Read the model definition and answer for the solid it produces. Units are mm, in the model's axes. A direction names the side the tool comes from. Coordinates: 2 decimals unless noted, no trailing zeros. Loops run counter-clockwise (first coordinate to the right, second up) from the corner with the lowest first, then second, coordinate; pieces in that order, holes last. Notation, with made-up numbers: (20.5, 86) -> (71.5, 86) arc R17 ccw to (71.5, 107) -> close; hole circle Ø9 at (-23, 43.5). An arc over 180 degrees is marked (long way). Answer as CSV lines item,"result".
```python
from build123d import *

# Parameters (mm, degrees)
SKETCH1_R           = 25.65
SKETCH1_R_2         = 16.9
SKETCH1_R_3         = 2.2
BOSS_EXTRUDE1_DEPTH = 3.1
SKETCH1_3_R         = 28.75
SKETCH1_3_R_2       = 25.65
BOSS_EXTRUDE2_DEPTH = 15
SKETCH2_R           = 2.2
BOSS_EXTRUDE4_DEPTH = 3.1


with BuildPart() as part:
    # Sketch1 → Boss-Extrude1 (new body)
    with BuildSketch(Plane(origin=(0, 0, 0), x_dir=(1, 0, 0), z_dir=(0, 1, 0))):
        Circle(SKETCH1_R)
        Circle(SKETCH1_R_2, mode=Mode.SUBTRACT)
        with Locations((0, 21.3)):
            Circle(SKETCH1_R_3, mode=Mode.SUBTRACT)
        with Locations((15.061374439, 15.061374439)):
            Circle(SKETCH1_R_3, mode=Mode.SUBTRACT)
        with Locations((21.3, 0)):
            Circle(SKETCH1_R_3, mode=Mode.SUBTRACT)
        with Locations((15.061374439, -15.061374439)):
            Circle(SKETCH1_R_3, mode=Mode.SUBTRACT)
        with Locations((0, -21.3)):
            Circle(SKETCH1_R_3, mode=Mode.SUBTRACT)
        with Locations((-15.061374439, -15.061374439)):
            Circle(SKETCH1_R_3, mode=Mode.SUBTRACT)
        with Locations((-21.3, 0)):
            Circle(SKETCH1_R_3, mode=Mode.SUBTRACT)
        with Locations((-15.061374439, 15.061374439)):
            Circle(SKETCH1_R_3, mode=Mode.SUBTRACT)
    extrude(amount=BOSS_EXTRUDE1_DEPTH)

    # Sketch1_3 → Boss-Extrude2 (add)
    with BuildSketch(Plane(origin=(0, 0, 0), x_dir=(1, 0, 0), z_dir=(0, 1, 0))):
        Circle(SKETCH1_3_R)
        Circle(SKETCH1_3_R_2, mode=Mode.SUBTRACT)
    extrude(amount=BOSS_EXTRUDE2_DEPTH)

    # Sketch2 → Boss-Extrude4 (add)
    with BuildSketch(Plane(origin=(0, 11.9, 0), x_dir=(1, 0, 0), z_dir=(0, 1, 0))):
        with BuildLine():
            ThreePointArc((25.65, 0), (25.555797131, 2.196299839), (25.273880469, 4.376467299))
            Line((25.273880469, 4.376467299), (20.845539906, 4.376467299))
            ThreePointArc((20.845539906, 4.376467299), (16.9, 0), (20.845539906, -4.376467299))
            Line((20.845539906, -4.376467299), (25.273880469, -4.376467299))
            ThreePointArc((25.273880469, -4.376467299), (25.555797131, -2.196299839), (25.65, 0))
        make_face()
        with Locations((21.3, 0)):
            Circle(SKETCH2_R, mode=Mode.SUBTRACT)
        with BuildLine():
            ThreePointArc((4.376467299, 25.273880469), (0, 25.65), (-4.376467299, 25.273880469))
            Line((-4.376467299, 25.273880469), (-4.376467299, 20.845539906))
            ThreePointArc((-4.376467299, 20.845539906), (0, 16.9), (4.376467299, 20.845539906))
            Line((4.376467299, 20.845539906), (4.376467299, 25.273880469))
        make_face()
        with Locations((0, 21.3)):
            Circle(SKETCH2_R, mode=Mode.SUBTRACT)
        with BuildLine():
            Line((-4.376467299, -20.845539906), (-4.376467299, -25.273880469))
            ThreePointArc((-4.376467299, -25.273880469), (0, -25.65), (4.376467299, -25.273880469))
            Line((4.376467299, -25.273880469), (4.376467299, -20.845539906))
            ThreePointArc((4.376467299, -20.845539906), (0, -16.9), (-4.376467299, -20.845539906))
        make_face()
        with Locations((0, -21.3)):
            Circle(SKETCH2_R, mode=Mode.SUBTRACT)
        with BuildLine():
            ThreePointArc((-20.845539906, -4.376467299), (-16.9, 0), (-20.845539906, 4.376467299))
            Line((-20.845539906, 4.376467299), (-25.273880469, 4.376467299))
            ThreePointArc((-25.273880469, 4.376467299), (-25.65, 0), (-25.273880469, -4.376467299))
            Line((-25.273880469, -4.376467299), (-20.845539906, -4.376467299))
        make_face()
        with Locations((-21.3, 0)):
            Circle(SKETCH2_R, mode=Mode.SUBTRACT)
    extrude(amount=BOSS_EXTRUDE4_DEPTH)


solid = part.part
```
Q1. Given pin 1 Ø5 at (x, y) = (6, 1.5) entering from +Z; pin 2 Ø1.5 at (x, y) = (-21, 10.5) entering from -Z; pin 3 Ø8 at (x, z) = (-3, -18) entering from +Y; pin 4 Ø2.5 at (y, z) = (14, 22.5) entering from +X, each flat-ended and moving along its own axis, determine where each tip first touches the part or whether it passes through.
Results:
pin 1,"stops at z = 28.54"
pin 2,"stops at z = -20.41"
pin 3,"stops at y = 15"
pin 4,"stops at x = 19.36"
Q2. For faces 1 (the face through (23, 13, -4.376)), 2 (the face through (17.16, 1.53, 14.4)), 3 (the face through (23, 11.9, 2)), determine the directions among +Z, -Z, +X, -X, +Y, -Y from which every point of the face is accessible in a straight line to the end or side of a thin tool.
Results:
face 1,"+Y"
face 2,"+Y, -Y"
face 3,"none"
Q3. A cutting plane is placed at D-D, the plane y = 5.75. Write down the section's boundary in (x, z).
Results:
outline,"circle Ø57.5 at (0, 0); hole circle Ø51.3 at (0, 0)"
Q4. For a pull along Y with two mould halves and no side action, classify faces 4 (the face through (-2.198, 1.528, -21.397)), 5 (the face through (23.694, 8.967, 9.824)), 6 (the face through (-17.2, 15, -0.1)) as pulls with the +Y half, pulls with the -Y half, needs draft (parallel to the pull), parting line crosses it, or undercut.
Results:
face 4,"needs draft"
face 5,"undercut"
face 6,"pulls with the +Y half"
Q5. Find the intervals of material crossed by probe 1 along Z at (x, y) = (0, 1.3); probe 2 along X at (y, z) = (13.05, 21.3), in increasing order. Write a range as [from, to].
Results:
probe 1,"z = [-28.75, -23.5], [-19.1, -16.9], [16.9, 19.1], [23.5, 28.75]"
probe 2,"x = [-19.31, -14.29], [-4.38, -2.2], [2.2, 4.38], [14.29, 19.31]"
Q6. A cutting plane is placed at A-A, the plane z = 0. Give the number of separate pieces and of enclosed holes in the cut face, and give its area (3 significant figures).
Results:
separate pieces,"6"
enclosed holes,"0"
area,"147 mm²"
